Geometry check sheet. Reference: the model listing, model coordinates, mm. Face numbers are marked on the shaded views. A direction names the side the tool comes from. Coordinates: 2 decimals unless noted, no trailing zeros. Order: outer loops, then holes, each group sorted by start corner. A loop starts at its lowest first (then second) coordinate and runs counter-clockwise, first axis right, second up. Notation, with made-up numbers: (75, 54) - (111, 54) arc R9 ccw to (111, 61) - close; hole circle Ø10 at (70.5, 88). An arc over 180 degrees is marked (long way). Return JSON: item names as keys, results as strings. Group by question number.
Item 1: Gauge pin test, flat ends, axial feed: pin 1 (0.5 mm diameter, centred on x = -89.5, z = -9, fed in from +Y); pin 2 (7 mm diameter, centred on x = -142.4, y = 0, fed in from +Z); pin 3 (4 mm diameter, centred on x = -42.4, y = 0, fed in from +Z); pin 4 (0.8 mm diameter, centred on x = -149, z = -9, fed in from -Y). Record the tip position at first contact, or that the pin passes through.
Item 2: Scan lines: probe 1 along Y at (x, z) = (-142.4, -0.75); probe 2 along X at (y, z) = (2, 8); probe 3 along Y at (x, z) = (-135, -7.25). Record each from-to range of solid material in increasing order.
Item 3: Section check B-B on y = 0. Enter the section's corners in (x, z).
Item 4: Tool access check on the marked faces 4 and 5. Record the directions out of +Z, -Z, +X, -X, +Y, -Y that give a thin tool (end or side, any length) a straight path to the whole face; none if there is none.
Item 5: Section check C-C on x = -106.5. Enter the section's corners in (y, z).
Item 6: Section check A-A on z = 2.5. Enter the section's corners in (x, y).
Item 7: Draft check along Y on the marked faces 1, 2 and 3. Enter one of: pulls with the +Y half, pulls with the -Y half, needs draft (parallel to the pull), parting line crosses it, or undercut.
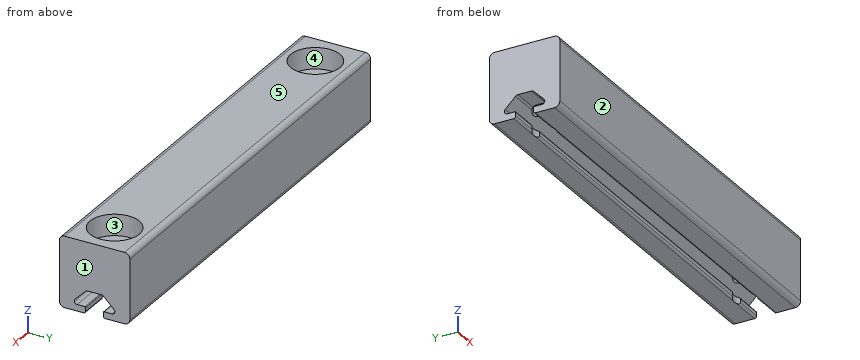
from build123d import *
from build123d.topology import SkipClean

# Parameters (mm, degrees)
BOSS_EXTRUDE1_DEPTH      = 152.4
BOSS_EXTRUDE1_DEPTH_BACK = 152.4
SKETCH4_R                = 2.15
BOSS_EXTRUDE2_DEPTH      = 95.2
SKETCH5_W                = 30
SKETCH5_H                = 30
CUT_EXTRUDE1_DEPTH       = 280
BOSS_EXTRUDE5_START      = -120
BOSS_EXTRUDE5_DEPTH      = 120
SKETCH9_R                = 3.15
CUT_EXTRUDE2_DEPTH       = 155.031685052
SKETCH10_R               = 7
CUT_EXTRUDE3_DEPTH       = 6


with BuildPart() as part:
    # Sketch3 → Boss-Extrude1 (new, two sides: drawn at the far end of the back side and taken through both)
    with BuildSketch(Plane(origin=(0, 0, 0), x_dir=(0, 0, -1), z_dir=(1, 0, 0)).offset(-BOSS_EXTRUDE1_DEPTH_BACK)):
        with BuildLine():
            Line((-5.515685425, 6.807463915), (-2.601114729, 3.892893219))
            ThreePointArc((-2.601114729, 3.892893219), (-2.27669138, 3.676120467), (-1.894007948, 3.6))
            Line((-1.894007948, 3.6), (0, 3.6))
            Line((0, 3.6), (0, 2.15))
            ThreePointArc((0, 2.15), (-1.52027958, 1.52027958), (-2.15, 0))
            Line((-2.15, 0), (-3.6, 0))
            Line((-3.6, 0), (-3.6, 1.894007948))
            ThreePointArc((-3.6, 1.894007948), (-3.676120467, 2.27669138), (-3.892893219, 2.601114729))
            Line((-3.892893219, 2.601114729), (-6.807463915, 5.515685425))
            ThreePointArc((-6.807463915, 5.515685425), (-7.679296086, 5.689103626), (-8.17314934, 4.95))
            Line((-8.17314934, 4.95), (-8.17314934, 2.7))
            ThreePointArc((-8.17314934, 2.7), (-8.231727984, 2.558578644), (-8.37314934, 2.5))
            Line((-8.37314934, 2.5), (-9.4, 2.5))
            ThreePointArc((-9.4, 2.5), (-9.824264069, 2.675735931), (-10, 3.1))
            Line((-10, 3.1), (-10, 8.5))
            ThreePointArc((-10, 8.5), (-9.560660172, 9.560660172), (-8.5, 10))
            Line((-8.5, 10), (-3.1, 10))
            ThreePointArc((-3.1, 10), (-2.675735931, 9.824264069), (-2.5, 9.4))
            Line((-2.5, 9.4), (-2.5, 8.37314934))
            ThreePointArc((-2.5, 8.37314934), (-2.558578644, 8.231727984), (-2.7, 8.17314934))
            Line((-2.7, 8.17314934), (-4.95, 8.17314934))
            ThreePointArc((-4.95, 8.17314934), (-5.689103626, 7.679296086), (-5.515685425, 6.807463915))
        make_face()
    extrude(amount=BOSS_EXTRUDE1_DEPTH + BOSS_EXTRUDE1_DEPTH_BACK)

    # Mirror1: part across plane


with BuildPart() as part_1:
    add(part.part)
    add(part.part.mirror(Plane.ZX))

    # Mirror2: part across plane


with BuildPart() as part_2:
    add(part_1.part)
    add(part_1.part.mirror(Plane.XY))

    # Sketch4 → Boss-Extrude2 (add)
    with SkipClean():  # the faces are left unmerged after this step: merging them gives an invalid solid
        with BuildSketch(Plane(origin=(152.4, 0, 0), x_dir=(0, 0, -1), z_dir=(1, 0, 0))):
            with BuildLine():
                Line((1.894007948, 3.6), (-1.894007948, 3.6))
                ThreePointArc((-1.894007948, 3.6), (-2.27669138, 3.676120467), (-2.601114729, 3.892893219))
                Line((-2.601114729, 3.892893219), (-5.515685425, 6.807463915))
                ThreePointArc((-5.515685425, 6.807463915), (-5.689103626, 7.679296086), (-4.95, 8.17314934))
                Line((-4.95, 8.17314934), (-2.7, 8.17314934))
                ThreePointArc((-2.7, 8.17314934), (-2.558578644, 8.231727984), (-2.5, 8.37314934))
                Line((-2.5, 8.37314934), (-2.5, 9.4))
                ThreePointArc((-2.5, 9.4), (-2.675735931, 9.824264069), (-3.1, 10))
                Line((-3.1, 10), (-8.5, 10))
                ThreePointArc((-8.5, 10), (-9.560660172, 9.560660172), (-10, 8.5))
                Line((-10, 8.5), (-10, 3.1))
                ThreePointArc((-10, 3.1), (-9.824264069, 2.675735931), (-9.4, 2.5))
                Line((-9.4, 2.5), (-8.37314934, 2.5))
                ThreePointArc((-8.37314934, 2.5), (-8.231727984, 2.558578644), (-8.17314934, 2.7))
                Line((-8.17314934, 2.7), (-8.17314934, 4.95))
                ThreePointArc((-8.17314934, 4.95), (-7.679296086, 5.689103626), (-6.807463915, 5.515685425))
                Line((-6.807463915, 5.515685425), (-3.892893219, 2.601114729))
                ThreePointArc((-3.892893219, 2.601114729), (-3.676120467, 2.27669138), (-3.6, 1.894007948))
                Line((-3.6, 1.894007948), (-3.6, -1.894007948))
                ThreePointArc((-3.6, -1.894007948), (-3.676120467, -2.27669138), (-3.892893219, -2.601114729))
                Line((-3.892893219, -2.601114729), (-6.807463915, -5.515685425))
                ThreePointArc((-6.807463915, -5.515685425), (-7.679296086, -5.689103626), (-8.17314934, -4.95))
                Line((-8.17314934, -4.95), (-8.17314934, -2.7))
                ThreePointArc((-8.17314934, -2.7), (-8.231727984, -2.558578644), (-8.37314934, -2.5))
                Line((-8.37314934, -2.5), (-9.4, -2.5))
                ThreePointArc((-9.4, -2.5), (-9.824264069, -2.675735931), (-10, -3.1))
                Line((-10, -3.1), (-10, -8.5))
                ThreePointArc((-10, -8.5), (-9.560660172, -9.560660172), (-8.5, -10))
                Line((-8.5, -10), (-3.1, -10))
                ThreePointArc((-3.1, -10), (-2.675735931, -9.824264069), (-2.5, -9.4))
                Line((-2.5, -9.4), (-2.5, -8.37314934))
                ThreePointArc((-2.5, -8.37314934), (-2.558578644, -8.231727984), (-2.7, -8.17314934))
                Line((-2.7, -8.17314934), (-4.95, -8.17314934))
                ThreePointArc((-4.95, -8.17314934), (-5.689103626, -7.679296086), (-5.515685425, -6.807463915))
                Line((-5.515685425, -6.807463915), (-2.601114729, -3.892893219))
                ThreePointArc((-2.601114729, -3.892893219), (-2.27669138, -3.676120467), (-1.894007948, -3.6))
                Line((-1.894007948, -3.6), (1.894007948, -3.6))
                ThreePointArc((1.894007948, -3.6), (2.27669138, -3.676120467), (2.601114729, -3.892893219))
                Line((2.601114729, -3.892893219), (5.515685425, -6.807463915))
                ThreePointArc((5.515685425, -6.807463915), (5.689103626, -7.679296086), (4.95, -8.17314934))
                Line((4.95, -8.17314934), (2.7, -8.17314934))
                ThreePointArc((2.7, -8.17314934), (2.558578644, -8.231727984), (2.5, -8.37314934))
                Line((2.5, -8.37314934), (2.5, -9.4))
                ThreePointArc((2.5, -9.4), (2.675735931, -9.824264069), (3.1, -10))
                Line((3.1, -10), (8.5, -10))
                ThreePointArc((8.5, -10), (9.560660172, -9.560660172), (10, -8.5))
                Line((10, -8.5), (10, -3.1))
                ThreePointArc((10, -3.1), (9.824264069, -2.675735931), (9.4, -2.5))
                Line((9.4, -2.5), (8.37314934, -2.5))
                ThreePointArc((8.37314934, -2.5), (8.231727984, -2.558578644), (8.17314934, -2.7))
                Line((8.17314934, -2.7), (8.17314934, -4.95))
                ThreePointArc((8.17314934, -4.95), (7.679296086, -5.689103626), (6.807463915, -5.515685425))
                Line((6.807463915, -5.515685425), (3.892893219, -2.601114729))
                ThreePointArc((3.892893219, -2.601114729), (3.676120467, -2.27669138), (3.6, -1.894007948))
                Line((3.6, -1.894007948), (3.6, 1.894007948))
                ThreePointArc((3.6, 1.894007948), (3.676120467, 2.27669138), (3.892893219, 2.601114729))
                Line((3.892893219, 2.601114729), (6.807463915, 5.515685425))
                ThreePointArc((6.807463915, 5.515685425), (7.679296086, 5.689103626), (8.17314934, 4.95))
                Line((8.17314934, 4.95), (8.17314934, 2.7))
                ThreePointArc((8.17314934, 2.7), (8.231727984, 2.558578644), (8.37314934, 2.5))
                Line((8.37314934, 2.5), (9.4, 2.5))
                ThreePointArc((9.4, 2.5), (9.824264069, 2.675735931), (10, 3.1))
                Line((10, 3.1), (10, 8.5))
                ThreePointArc((10, 8.5), (9.560660172, 9.560660172), (8.5, 10))
                Line((8.5, 10), (3.1, 10))
                ThreePointArc((3.1, 10), (2.675735931, 9.824264069), (2.5, 9.4))
                Line((2.5, 9.4), (2.5, 8.37314934))
                ThreePointArc((2.5, 8.37314934), (2.558578644, 8.231727984), (2.7, 8.17314934))
                Line((2.7, 8.17314934), (4.95, 8.17314934))
                ThreePointArc((4.95, 8.17314934), (5.689103626, 7.679296086), (5.515685425, 6.807463915))
                Line((5.515685425, 6.807463915), (2.601114729, 3.892893219))
                ThreePointArc((2.601114729, 3.892893219), (2.27669138, 3.676120467), (1.894007948, 3.6))
            make_face()
            Circle(SKETCH4_R, mode=Mode.SUBTRACT)
        extrude(amount=BOSS_EXTRUDE2_DEPTH)

    # Sketch5 → Cut-Extrude1 (cut)
    with BuildSketch(Plane(origin=(247.6, 0, 0), x_dir=(0, 0, -1), z_dir=(1, 0, 0))):
        Rectangle(SKETCH5_W, SKETCH5_H)
    extrude(amount=-CUT_EXTRUDE1_DEPTH, mode=Mode.SUBTRACT)

    # Sketch8 → Boss-Extrude5 (add)
    with BuildSketch(Plane(origin=(-32.4, 0, 0), x_dir=(0, 0, -1), z_dir=(1, 0, 0)).offset(BOSS_EXTRUDE5_START)):
        with BuildLine():
            Line((-8.5, 10), (8.5, 10))
            ThreePointArc((8.5, 10), (9.560660172, 9.560660172), (10, 8.5))
            Line((10, 8.5), (10, 3.1))
            ThreePointArc((10, 3.1), (9.824264069, 2.675735931), (9.4, 2.5))
            Line((9.4, 2.5), (8.37314934, 2.5))
            ThreePointArc((8.37314934, 2.5), (8.231727984, 2.558578644), (8.17314934, 2.7))
            Line((8.17314934, 2.7), (8.17314934, 4.95))
            ThreePointArc((8.17314934, 4.95), (7.679296086, 5.689103626), (6.807463915, 5.515685425))
            Line((6.807463915, 5.515685425), (3.892893219, 2.601114729))
            ThreePointArc((3.892893219, 2.601114729), (3.676120467, 2.27669138), (3.6, 1.894007948))
            Line((3.6, 1.894007948), (3.6, -1.894007948))
            ThreePointArc((3.6, -1.894007948), (3.676120467, -2.27669138), (3.892893219, -2.601114729))
            Line((3.892893219, -2.601114729), (6.807463915, -5.515685425))
            ThreePointArc((6.807463915, -5.515685425), (7.679296086, -5.689103626), (8.17314934, -4.95))
            Line((8.17314934, -4.95), (8.17314934, -2.7))
            ThreePointArc((8.17314934, -2.7), (8.231727984, -2.558578644), (8.37314934, -2.5))
            Line((8.37314934, -2.5), (9.4, -2.5))
            ThreePointArc((9.4, -2.5), (9.824264069, -2.675735931), (10, -3.1))
            Line((10, -3.1), (10, -8.5))
            ThreePointArc((10, -8.5), (9.560660172, -9.560660172), (8.5, -10))
            Line((8.5, -10), (-8.5, -10))
            ThreePointArc((-8.5, -10), (-9.560660172, -9.560660172), (-10, -8.5))
            Line((-10, -8.5), (-10, 8.5))
            ThreePointArc((-10, 8.5), (-9.560660172, 9.560660172), (-8.5, 10))
        make_face()
    extrude(amount=BOSS_EXTRUDE5_DEPTH)

    # Sketch9 → Cut-Extrude2 (cut, through all)
    with BuildSketch(Plane.XY.offset(10)):
        with Locations((-142.4, 0)):
            Circle(SKETCH9_R)
        with Locations((-42.4, 0)):
            Circle(SKETCH9_R)
    extrude(amount=-CUT_EXTRUDE2_DEPTH, mode=Mode.SUBTRACT)

    # Sketch10 → Cut-Extrude3 (cut)
    with BuildSketch(Plane.XY.offset(10)):
        with Locations((-142.4, 0)):
            Circle(SKETCH10_R)
        with Locations((-42.4, 0)):
            Circle(SKETCH10_R)
    extrude(amount=-CUT_EXTRUDE3_DEPTH, mode=Mode.SUBTRACT)


solid = part_2.part
Computed:
{
 "1": {"pin 1": "stops at y = 9.98", "pin 2": "stops at z = 4", "pin 3": "passes through", "pin 4": "stops at y = -10"},
 "2": {"probe 1": "y = -10 to -3.15, 3.15 to 10", "probe 2": "x = -152.4 to -149.11, -135.69 to -49.11, -35.69 to -32.4", "probe 3": "y = -10 to -5.74, 5.74 to 10"},
 "3": {"outline": "(-152.4, -3.6) - (-145.55, -3.6) - (-145.55, 4) - (-149.4, 4) - (-149.4, 10) - (-152.4, 10) - close; (-139.25, -3.6) - (-45.55, -3.6) - (-45.55, 4) - (-49.4, 4) - (-49.4, 10) - (-135.4, 10) - (-135.4, 4) - (-139.25, 4) - close; (-39.25, -3.6) - (-32.4, -3.6) - (-32.4, 10) - (-35.4, 10) - (-35.4, 4) - (-39.25, 4) - close"},
 "4": {"face 4": "+Z", "face 5": "+Z, +X, -X, +Y, -Y"},
 "5": {"outline": "(-10, -8.5) arc R1.5 ccw to (-8.5, -10) - (-3.1, -10) arc R0.6 ccw to (-2.5, -9.4) - (-2.5, -8.37) arc R0.2 ccw to (-2.7, -8.17) - (-4.95, -8.17) arc R0.8 cw to (-5.52, -6.81) - (-2.6, -3.89) arc R1 cw to (-1.89, -3.6) - (1.89, -3.6) arc R1 cw to (2.6, -3.89) - (5.52, -6.81) arc R0.8 cw to (4.95, -8.17) - (2.7, -8.17) arc R0.2 ccw to (2.5, -8.37) - (2.5, -9.4) arc R0.6 ccw to (3.1, -10) - (8.5, -10) arc R1.5 ccw to (10, -8.5) - (10, 8.5) arc R1.5 ccw to (8.5, 10) - (-8.5, 10) arc R1.5 ccw to (-10, 8.5) - close"},
 "6": {"outline": "(-152.4, -10) - (-32.4, -10) - (-32.4, 10) - (-152.4, 10) - close; hole circle Ø6.3 at (-142.4, 0); hole circle Ø6.3 at (-42.4, 0)"},
 "7": {"face 1": "needs draft", "face 2": "pulls with the -Y half", "face 3": "undercut"}
}
